CAD build for the part. Positions are in the model's coordinates, mm. Face numbers are marked on the shaded views. A direction names the side the tool comes from. Give positions to 0.01 mm unless a question says otherwise; leave off trailing zeros. Loops run counter-clockwise (first coordinate to the right, second up) from the corner with the lowest first, then second, coordinate; pieces in that order, holes last. Notation, with made-up numbers: (60, -18) -> (72, -18) arc R20 ccw to (72, 19) -> close; hole circle Ø7 at (54.5, -16). An arc over 180 degrees is marked (long way). Use one line per item in the form item = value.
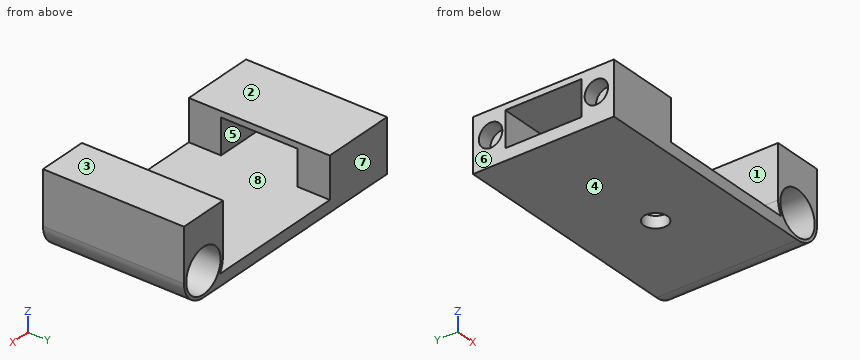
```python
from build123d import *

# Parameters (mm, degrees)
SKETCH_R           = 7.5
PAD_DEPTH          = 24
SKETCH001_R        = 4
POCKET_DEPTH       = 5
POLARPATTERN_COUNT = 2
SKETCH002_W        = 12
SKETCH002_H        = 26
POCKET001_DEPTH    = 25
SKETCH004_R        = 4
POCKET002_DEPTH    = 5


with BuildPart() as part:
    # Sketch → Pad (new body, symmetric)
    with BuildSketch(Plane.XZ):
        with BuildLine():
            Line((-49, 18), (-49, 0))
            Line((-49, 0), (31.211103, 0))
            ThreePointArc((31.211103, 0), (37.22151, 2.489592), (39.711103, 8.5))
            Line((39.711103, 26.499979), (39.711103, 8.5))
            Line((22.711103, 26.499979), (39.711103, 26.499979))
            Line((22.711103, 8.499979), (22.711103, 26.499979))
            ThreePointArc((22.711103, 8.499979), (23.03968, 6.159517), (24, 4))
            Line((-24, 4), (24, 4))
            Line((-24, 18), (-24, 4))
            Line((-49, 18), (-24, 18))
        make_face()
        with Locations((31.211103, 8.5)):
            Circle(SKETCH_R, mode=Mode.SUBTRACT)
    extrude(amount=PAD_DEPTH, both=True)

    # Sketch001 → Pocket (cut)
    with BuildSketch(Plane(origin=(0, 0, 4), x_dir=(-1, 0, 0), z_dir=(0, 0, 1))):
        Circle(SKETCH001_R)
    pocket = extrude(amount=-POCKET_DEPTH, mode=Mode.SUBTRACT)

    # PolarPattern: Pocket ×2 about axis
    polarpattern_axis = Axis((0, 0, 4), (0, 0, 1))
    for i in range(1, POLARPATTERN_COUNT):
        add(pocket.rotate(polarpattern_axis, i * 360 / POLARPATTERN_COUNT), mode=Mode.SUBTRACT)

    # Sketch002 → Pocket001 (cut)
    with BuildSketch(Plane(origin=(-49, 0, 0), x_dir=(0, 0, -1), z_dir=(-1, 0, 0))):
        with Locations((-10, 0)):
            Rectangle(SKETCH002_W, SKETCH002_H)
    extrude(amount=-POCKET001_DEPTH, mode=Mode.SUBTRACT)

    # Sketch004 → Pocket002 (cut)
    with BuildSketch(Plane(origin=(-49, 0, 0), x_dir=(0, 0, -1), z_dir=(-1, 0, 0))):
        with Locations((-10, -18)):
            Circle(SKETCH004_R)
        with Locations((-10, 18)):
            Circle(SKETCH004_R)
    extrude(amount=-POCKET002_DEPTH, mode=Mode.SUBTRACT)


solid = part.part
```
1. Cut at D-D, the plane y = -18. Write the cut outline in (x, z), then the cut area to 3 significant figures.
Result sheet:
outline = (-49, 0) -> (31.21, 0) arc R8.5 ccw to (39.71, 8.5) -> (39.71, 26.5) -> (22.71, 26.5) -> (22.71, 8.5) arc R8.5 ccw to (24, 4) -> (-24, 4) -> (-24, 18) -> (-49, 18) -> (-49, 14) -> (-44, 14) -> (-44, 6) -> (-49, 6) -> close; hole circle Ø15 at (31.21, 8.5)
area = 853 mm^2
2. Cut at C-C, the plane z = 10.75. Write the cut outline in (x, y), then the cut area to 3 significant figures.
Result sheet:
outline = (-49, -24) -> (-24, -24) -> (-24, -13) -> (-49, -13) -> (-49, -14.07) -> (-44, -14.07) -> (-44, -21.93) -> (-49, -21.93) -> close; (-49, 13) -> (-24, 13) -> (-24, 24) -> (-49, 24) -> (-49, 21.93) -> (-44, 21.93) -> (-44, 14.07) -> (-49, 14.07) -> close; (22.71, -24) -> (24.06, -24) -> (24.06, 24) -> (22.71, 24) -> close; (38.37, -24) -> (39.71, -24) -> (39.71, 24) -> (38.37, 24) -> close
area = 601 mm^2
3. Cut at A-A, the plane y = 0. Write the cut outline in (x, z).
Result sheet:
outline = (-49, 0) -> (-4, 0) -> (-4, 4) -> (-49, 4) -> close; (-49, 16) -> (-24, 16) -> (-24, 18) -> (-49, 18) -> close; (4, 0) -> (31.21, 0) arc R8.5 ccw to (39.71, 8.5) -> (39.71, 26.5) -> (22.71, 26.5) -> (22.71, 8.5) arc R8.5 ccw to (24, 4) -> (4, 4) -> close; hole circle Ø15 at (31.21, 8.5)
4. Mould opens along Y. For the marked faces 6, 7 and 8 say: pulls with the +Y half, pulls with the -Y half, needs draft (parallel to the pull), parting line crosses it, or undercut.
Result sheet:
face_6 = needs draft
face_7 = pulls with the +Y half
face_8 = undercut
5. Cut at B-B, the plane y = -7. Write the cut outline in (x, z).
Result sheet:
outline = (-49, 0) -> (31.21, 0) arc R8.5 ccw to (39.71, 8.5) -> (39.71, 26.5) -> (22.71, 26.5) -> (22.71, 8.5) arc R8.5 ccw to (24, 4) -> (-49, 4) -> close; (-49, 16) -> (-24, 16) -> (-24, 18) -> (-49, 18) -> close; hole circle Ø15 at (31.21, 8.5)
6. Drill centre lines: line 1 (Y direction, x = -45, z = 10); line 2 (X direction, y = -16.5, z = 16.75); line 3 (X direction, y = 16.5, z = 6.5). Where is each one in solid material? Low to high.
Result sheet:
line_1 = -24 to -22, -14 to -13, 13 to 14, 22 to 24
line_2 = -49 to -24, 22.71 to 39.71
line_3 = -44 to -24, 22.95 to 23.98, 38.44 to 39.47
7. Tool access for the marked faces 1, 2, 3, 4 and 5: list every direction of +Z, -Z, +X, -X, +Y, -Y with a clear straight run to the whole face (end or side of a thin tool).
Result sheet:
face_1 = +Z, +Y, -Y
face_2 = +Z, -X, +Y, -Y
face_3 = +Z, +X, -X, +Y, -Y
face_4 = -Z, +X, -X, +Y, -Y
face_5 = -X
8. Drop flat-ended pins along their axis: P1, Ø2.5, axis at y = -19.5, z = 9.5, coming from the -X side; P2, Ø10.5, axis at x = 0, y = 0, coming from the +Z side; P3, Ø2, axis at y = 3, z = 7.5, coming from the -X side. Give the stop position or say it passes through.
Result sheet:
P1 = -44
P2 = 4
P3 = 22.71
